```python
from build123d import *

# Parameters (mm, degrees)
SKETCH1_W                 = 140
SKETCH1_H                 = 100
BOSS_EXTRUDE1_DEPTH       = 3
SKETCH3_W                 = 16
SKETCH3_H                 = 100
BOSS_EXTRUDE2_DEPTH       = 2.5
SKETCH4_W                 = 12.5
SKETCH4_H                 = 5.5
CUT_EXTRUDE1_DEPTH        = 1.5
LPATTERN1_COUNT           = 4
LPATTERN1_PITCH           = 30
LPATTERN1_COPY_1_SKETCH_W = 12.5
LPATTERN1_COPY_1_SKETCH_H = 5.5
LPATTERN1_COPY_1_DEPTH    = 1.5
LPATTERN1_COPY_2_SKETCH_W = 12.5
LPATTERN1_COPY_2_SKETCH_H = 5.5
LPATTERN1_COPY_2_DEPTH    = 1.5
LPATTERN1_COPY_3_SKETCH_W = 12.5
LPATTERN1_COPY_3_SKETCH_H = 5.5
LPATTERN1_COPY_3_DEPTH    = 1.5
CUT_EXTRUDE3_DEPTH        = 123.102416029
CUT_EXTRUDE3_DEPTH_BACK   = 123.102416029
SKETCH6_W                 = 0.2
SKETCH6_H                 = 3
CUT_EXTRUDE5_DEPTH        = 1.5
LPATTERN2_COUNT           = 2
LPATTERN2_PITCH           = 30
LPATTERN2_COL_COUNT       = 2
LPATTERN2_COL_PITCH       = 30
MIRROR4_COPY_1_DEPTH      = 1.5
MIRROR4_COPY_2_DEPTH      = 1.5
SKETCH13_W                = 1
SKETCH13_H                = 40
SKETCH13_H_2              = 36
CUT_EXTRUDE7_DEPTH        = 10
SKETCH15_W                = 80
SKETCH15_H                = 3
BOSS_EXTRUDE4_DEPTH       = 10
FILLET2_R                 = 5
FILLET3_R                 = 3
SKETCH17_W                = 12.35
SKETCH17_H                = 2.25
CUT_EXTRUDE9_DEPTH        = 1.5
SKETCH18_R                = 1.6
CUT_EXTRUDE10_DEPTH       = 10
CUT_EXTRUDE11_DEPTH       = 10
SKETCH25_W                = 42.063690351
SKETCH25_H                = 4.970755329
CUT_EXTRUDE12_DEPTH       = 10


with BuildPart() as part:
    # Sketch1 → Boss-Extrude1 (new body)
    with BuildSketch(Plane.XY):
        Rectangle(SKETCH1_W, SKETCH1_H)
    extrude(amount=BOSS_EXTRUDE1_DEPTH)

    # Sketch3 → Boss-Extrude2 (add)
    with BuildSketch(Plane(origin=(0, 0, 0), x_dir=(-1, 0, 0), z_dir=(0, 0, -1))):
        with Locations((-60, 0)):
            Rectangle(SKETCH3_W, SKETCH3_H)
        with Locations((60, 0)):
            Rectangle(SKETCH3_W, SKETCH3_H)
    extrude(amount=BOSS_EXTRUDE2_DEPTH)

    # Sketch4 → Cut-Extrude1 (cut)
    with BuildSketch(Plane(origin=(0, 0, -2.5), x_dir=(-1, 0, 0), z_dir=(0, 0, -1))):
        with Locations((-60, 45)):
            Rectangle(SKETCH4_W, SKETCH4_H)
    cut_extrude1 = extrude(amount=-CUT_EXTRUDE1_DEPTH, mode=Mode.SUBTRACT)

    # Mirror1: Cut-Extrude1 across plane
    add(cut_extrude1.mirror(Plane(origin=(0, 0, 0), x_dir=(0, 0, 1), z_dir=(1, 0, 0))), mode=Mode.SUBTRACT)

    # LPattern1: Cut-Extrude1 ×4
    with Locations(*[(0, -i * LPATTERN1_PITCH, 0) for i in range(1, LPATTERN1_COUNT)]):
        add(cut_extrude1, mode=Mode.SUBTRACT)

    # LPattern1 copy 1 sketch → LPattern1 copy 1 (cut)
    with BuildSketch(Plane(origin=(0, -30, -2.5), x_dir=(1, 0, 0), z_dir=(0, 0, -1))):
        with Locations((-60, -45)):
            Rectangle(LPATTERN1_COPY_1_SKETCH_W, LPATTERN1_COPY_1_SKETCH_H)
    extrude(amount=-LPATTERN1_COPY_1_DEPTH, mode=Mode.SUBTRACT)

    # LPattern1 copy 2 sketch → LPattern1 copy 2 (cut)
    with BuildSketch(Plane(origin=(0, -60, -2.5), x_dir=(1, 0, 0), z_dir=(0, 0, -1))):
        with Locations((-60, -45)):
            Rectangle(LPATTERN1_COPY_2_SKETCH_W, LPATTERN1_COPY_2_SKETCH_H)
    extrude(amount=-LPATTERN1_COPY_2_DEPTH, mode=Mode.SUBTRACT)

    # LPattern1 copy 3 sketch → LPattern1 copy 3 (cut)
    with BuildSketch(Plane(origin=(0, -90, -2.5), x_dir=(1, 0, 0), z_dir=(0, 0, -1))):
        with Locations((-60, -45)):
            Rectangle(LPATTERN1_COPY_3_SKETCH_W, LPATTERN1_COPY_3_SKETCH_H)
    extrude(amount=-LPATTERN1_COPY_3_DEPTH, mode=Mode.SUBTRACT)

    # Sketch6 → Cut-Extrude3 (cut, two sides: drawn at the far end of the back side and taken through both)
    with BuildSketch(Plane(origin=(0, 50, 0), x_dir=(1, 0, 0), z_dir=(0, 1, 0)).offset(-CUT_EXTRUDE3_DEPTH_BACK)):
        with Locations((-69.9, -1.5)):
            Rectangle(SKETCH6_W, SKETCH6_H)
        with Locations((69.9, -1.5)):
            Rectangle(SKETCH6_W, SKETCH6_H)
    extrude(amount=CUT_EXTRUDE3_DEPTH + CUT_EXTRUDE3_DEPTH_BACK, mode=Mode.SUBTRACT)

    # Sketch11 → Cut-Extrude5 (cut)
    with BuildSketch(Plane(origin=(0, 0, -2.5), x_dir=(-1, 0, 0), z_dir=(0, 0, -1))):
        Polygon((-53.75, 12.25), (-60, -7.75), (-66.25, 12.25), align=None)
    cut_extrude5 = extrude(amount=-CUT_EXTRUDE5_DEPTH, mode=Mode.SUBTRACT)

    # LPattern2: Cut-Extrude5 ×2
    with Locations(*[(0, i * LPATTERN2_PITCH, 0) for i in range(1, LPATTERN2_COUNT)]):
        add(cut_extrude5, mode=Mode.SUBTRACT)

    # LPattern2 col: Cut-Extrude5 ×2
    with Locations(*[(0, -i * LPATTERN2_COL_PITCH, 0) for i in range(1, LPATTERN2_COL_COUNT)]):
        add(cut_extrude5, mode=Mode.SUBTRACT)

    # Mirror4: Cut-Extrude5 across plane
    add(cut_extrude5.mirror(Plane(origin=(0, 0, 0), x_dir=(0, 0, 1), z_dir=(1, 0, 0))), mode=Mode.SUBTRACT)

    # Mirror4 copy 1 sketch → Mirror4 copy 1 (cut)
    with BuildSketch(Plane(origin=(0, 30, -2.5), x_dir=(1, 0, 0), z_dir=(0, 0, -1))):
        Polygon((-53.75, -12.25), (-60, 7.75), (-66.25, -12.25), align=None)
    extrude(amount=-MIRROR4_COPY_1_DEPTH, mode=Mode.SUBTRACT)

    # Mirror4 copy 2 sketch → Mirror4 copy 2 (cut)
    with BuildSketch(Plane(origin=(0, -30, -2.5), x_dir=(1, 0, 0), z_dir=(0, 0, -1))):
        Polygon((-53.75, -12.25), (-60, 7.75), (-66.25, -12.25), align=None)
    extrude(amount=-MIRROR4_COPY_2_DEPTH, mode=Mode.SUBTRACT)

    # Sketch13 → Cut-Extrude7 (cut)
    with BuildSketch(Plane(origin=(0, 0, 0), x_dir=(-1, 0, 0), z_dir=(0, 0, -1))):
        with Locations((-46.5, 25)):
            Rectangle(SKETCH13_W, SKETCH13_H)
        with Locations((-46.5, -23)):
            Rectangle(SKETCH13_W, SKETCH13_H_2)
    cut_extrude7 = extrude(amount=-CUT_EXTRUDE7_DEPTH, mode=Mode.SUBTRACT)

    # Mirror7: Cut-Extrude7 across plane
    add(cut_extrude7.mirror(Plane(origin=(0, 0, 0), x_dir=(0, 0, 1), z_dir=(1, 0, 0))), mode=Mode.SUBTRACT)

    # Sketch15 → Boss-Extrude4 (add)
    with BuildSketch(Plane(origin=(0, 0, 0), x_dir=(-1, 0, 0), z_dir=(0, 0, -1))):
        with Locations((0, 48.5)):
            Rectangle(SKETCH15_W, SKETCH15_H)
    extrude(amount=BOSS_EXTRUDE4_DEPTH)

    # Fillet2
    fillet2_edges = [part.edges().sort_by_distance(p)[0] for p in [
        (40, 48.5, -10),
        (-40, 48.5, -10),
    ]]
    fillet(fillet2_edges, radius=FILLET2_R)

    # Fillet3
    fillet3_edges = [part.edges().sort_by_distance(p)[0] for p in [
        (0, 47, 0),
    ]]
    fillet(fillet3_edges, radius=FILLET3_R)

    # Sketch17 → Cut-Extrude9 (cut)
    with BuildSketch(Plane(origin=(0, 0, -2.5), x_dir=(-1, 0, 0), z_dir=(0, 0, -1))):
        with Locations((-60.075, -48.875)):
            Rectangle(SKETCH17_W, SKETCH17_H)
    cut_extrude9 = extrude(amount=-CUT_EXTRUDE9_DEPTH, mode=Mode.SUBTRACT)

    # Mirror8: Cut-Extrude9 across plane
    add(cut_extrude9.mirror(Plane(origin=(0, 0, 0), x_dir=(0, 0, 1), z_dir=(1, 0, 0))), mode=Mode.SUBTRACT)

    # Sketch18 → Cut-Extrude10 (cut)
    with BuildSketch(Plane(origin=(0, 50, 0), x_dir=(1, 0, 0), z_dir=(0, 1, 0))):
        with Locations(Location((-25, 3, 0), (0, 0, 180))):
            Circle(SKETCH18_R)
        with Locations(Location((25, 3, 0), (0, 0, 180))):
            Circle(SKETCH18_R)
    extrude(amount=-CUT_EXTRUDE10_DEPTH, mode=Mode.SUBTRACT)

    # Sketch24 → Cut-Extrude11 (cut)
    with BuildSketch(Plane.XY.offset(3)):
        with BuildLine():
            Line((-24.07859083, -40.000422033), (-24.07859083, -43.681991466))
            ThreePointArc((-24.07859083, -43.681991466), (-23.20025424, -45.92649129), (-21.031820585, -46.978703301))
            ThreePointArc((-21.031820585, -46.978703301), (-16.771632398, -47.280714447), (-12.507162767, -47.514622336))
            Line((-12.507162767, -47.514622336), (12.507211948, -47.514622336))
            ThreePointArc((12.507211948, -47.514622336), (16.771681578, -47.280714447), (21.031869766, -46.978703301))
            ThreePointArc((21.031869766, -46.978703301), (23.20030342, -45.92649129), (24.078640011, -43.681991466))
            Line((24.078640011, -43.681991466), (24.078640011, -40.000422033))
            ThreePointArc((24.078640011, -40.000422033), (25.579081322, -36.061125654), (29.320000625, -34.118214731))
            ThreePointArc((29.320000625, -34.118214731), (34.297548475, -33.493160314), (39.26185403, -32.770425237))
            ThreePointArc((39.26185403, -32.770425237), (42.306988396, -0.000422033), (39.26185403, 32.769581172))
            ThreePointArc((39.26185403, 32.769581172), (37.111227515, 33.094915187), (34.957907382, 33.401915241))
            Line((34.957907382, 33.401915241), (34.886534309, 32.907026835))
            ThreePointArc((34.886534309, 32.907026835), (2.459e-05, 35.306541773), (-34.886485128, 32.907026835))
            Line((-34.886485128, 32.907026835), (-34.957858201, 33.401915241))
            ThreePointArc((-34.957858201, 33.401915241), (-37.111178334, 33.094915187), (-39.261804849, 32.769581172))
            ThreePointArc((-39.261804849, 32.769581172), (-42.306939215, -0.000422033), (-39.261804849, -32.770425237))
            ThreePointArc((-39.261804849, -32.770425237), (-34.297499295, -33.493160314), (-29.319951444, -34.118214731))
            ThreePointArc((-29.319951444, -34.118214731), (-25.579032142, -36.061125654), (-24.07859083, -40.000422033))
        make_face()
    extrude(amount=-CUT_EXTRUDE11_DEPTH, mode=Mode.SUBTRACT)

    # Sketch25 → Cut-Extrude12 (cut)
    with BuildSketch(Plane(origin=(0, 0, 0), x_dir=(-1, 0, 0), z_dir=(0, 0, -1))):
        with Locations((-2.459e-05, -47.514622336)):
            Rectangle(SKETCH25_W, SKETCH25_H)
    extrude(amount=-CUT_EXTRUDE12_DEPTH, mode=Mode.SUBTRACT)


solid = part.part
```
Read the model definition and answer for the solid it produces. Units are mm, in the model's axes. A direction names the side the tool comes from. Coordinates: 2 decimals unless noted, no trailing zeros. Write each loop counter-clockwise with the first axis right and the second up, starting at its lowest first coordinate (ties: lowest second). Pieces come first, ordered by that corner, then holes. Notation, with made-up numbers: (15.25, 54) -> (34.25, 54) arc R13 ccw to (34.25, 72) -> close; hole circle Ø4 at (29.25, 47). An arc over 180 degrees is marked (long way). Write item = value, one per line.
(1) Straight lines are drawn through the part: L1, parallel to Z at x = 25, y = 47.8; L2, parallel to X at y = -32.5, z = 1.25; L3, parallel to X at y = -26, z = -0.75. For each, find the intervals that lie inside material, in ascending order. Write a range as from..to.
From the geometry:
L1 = -10..-4.6, -1.4..3
L2 = -69.8..-47, -46..-39.31, 39.31..46, 47..69.8
L3 = -68..-52, 52..68
(2) Section A-A on y = -29 is taken. Count the separate pieces of the cut face and the enclosed holes in it, plus the area to 3 significant figures.
From the geometry:
separate_pieces = 4
enclosed_holes = 0
area = 237 mm2
(3) Given pin 1 Ø0.8 at (y, z) = (-45.5, -2) entering from +X; pin 2 Ø1.4 at (x, y) = (69, 21) entering from -Z; pin 3 Ø5 at (y, z) = (11, -7) entering from +X; pin 4 Ø4 at (y, z) = (46.5, -3.5) entering from -X, each flat-ended and moving along its own axis, determine where each tip first touches the part or whether it passes through.
From the geometry:
pin_1 = 68
pin_2 = 0
pin_3 = through
pin_4 = -68
(4) For a pull along X with two mould halves and no side action, classify faces 4 (the face through (37.14, 33.09, 1.52)), 5 (the face through (0, 49, -10)), 6 (the face through (39, 49, -8)) as +X half, -X half, draft (parallel to the pull), parting line (faces both ways), or undercut.
From the geometry:
face_4 = undercut
face_5 = draft
face_6 = +X half
(5) Which of the six approach directions +Z, -Z, +X, -X, +Y, -Y give full straight-line access (tool end or side, diameter ignored) to faces 1 (the face through (-56.83, 32.39, -1.76)), 2 (the face through (21.032, -49, 1)), 3 (the face through (40, 48, -2))?
From the geometry:
face_1 = -Z
face_2 = +Z, -Z, -Y
face_3 = -Z, +Y, -Y
(6) Section B-B on x = 33 is taken. Write down the section's boundary in (y, z), plus the area to 3 significant figures.
From the geometry:
outline = (-50, 0) -> (-33.67, 0) -> (-33.67, 3) -> (-50, 3) -> close; (33.16, 0) -> (44, 0) arc R3 cw to (47, -3) -> (47, -10) -> (50, -10) -> (50, 3) -> (33.16, 3) -> close
area = 131 mm2
(7) Section D-D on x = 19 is taken. Write down the section's boundary in (y, z), plus the area to 3 significant figures.
From the geometry:
outline = (34.6, 0) -> (44, 0) arc R3 cw to (47, -3) -> (47, -10) -> (50, -10) -> (50, 3) -> (34.6, 3) -> close
area = 78.1 mm2
